```python
from build123d import *

# Parameters (mm, degrees)
F0_R     = 12.7
F1_DEPTH = 12.7
F3_R     = 4.7625
F3_R_2   = 2.7305
F4_DEPTH = 6.35


with BuildPart() as f1:
    # F0 (on Top) → F1 (new body)
    with BuildSketch(Plane.XY):
        Circle(F0_R)
    extrude(amount=F1_DEPTH)

    # F3 (on offset) → F4 (join)
    with BuildSketch(Plane.XY.offset(12.7)):
        with Locations((-5.399791, 5.753814)):
            Circle(F3_R)
        with Locations((-5.399791, 5.753814)):
            Circle(F3_R_2, mode=Mode.SUBTRACT)
        with Locations((-5.753814, -5.399791)):
            Circle(F3_R)
        with Locations((-5.753814, -5.399791)):
            Circle(F3_R_2, mode=Mode.SUBTRACT)
        with Locations((5.399791, -5.753814)):
            Circle(F3_R)
        with Locations((5.399791, -5.753814)):
            Circle(F3_R_2, mode=Mode.SUBTRACT)
        with Locations((5.753814, 5.399791)):
            Circle(F3_R)
        with Locations((5.753814, 5.399791)):
            Circle(F3_R_2, mode=Mode.SUBTRACT)
    extrude(amount=F4_DEPTH)


solid = f1.part
```
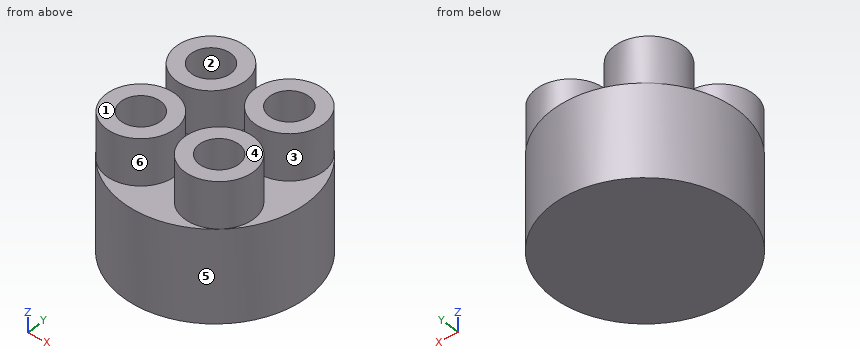
CAD build for the part. Positions are in the model's coordinates, mm. Face numbers are marked on the shaded views. A direction names the side the tool comes from. Coordinates: 2 decimals unless noted, no trailing zeros. Order: outer loops, then holes, each group sorted by start corner. A loop starts at its lowest first (then second) coordinate and runs counter-clockwise, first axis right, second up.
(1) Saw through at A-A, the plane x = -7.5. Write the cut outline in (y, z).
Solution:
outline: (-10.25, 0) - (10.25, 0) - (10.25, 12.7) - (10.03, 12.7) - (10.03, 19.05) - (7.5, 19.05) - (7.5, 12.7) - (4.01, 12.7) - (4.01, 19.05) - (1.48, 19.05) - (1.48, 12.7) - (-0.97, 12.7) - (-0.97, 19.05) - (-3.3, 19.05) - (-3.3, 12.7) - (-7.5, 12.7) - (-7.5, 19.05) - (-9.83, 19.05) - (-9.83, 12.7) - (-10.25, 12.7) - close
(2) Which spindle directions (+Z, -Z, +X, -X, +Y, -Y) get a long thin tool onto all of the face, cutting with end or side? Do the marked faces 1 and 2. Say none if no direction does.
Solution:
face 1: +Z, +X, -X, +Y, -Y
face 2: +Z
(3) Saw through at C-C, the plane z = 12.25. Write the cut outline in (x, y).
Solution:
outline: circle Ø25.4 at (0, 0)
(4) Mould opens along Y. For the marked faces 3, 4, 5 and 6 say: released by +Y, released by -Y, zero draft, split by the parting line, or undercut.
Solution:
face 3: undercut
face 4: zero draft
face 5: split by the parting line
face 6: undercut
(5) Saw through at B-B, the plane y = 9.5. Write the cut outline in (x, z).
Solution:
outline: (-8.43, 0) - (8.43, 0) - (8.43, 12.7) - (8.18, 12.7) - (8.18, 19.05) - (3.33, 19.05) - (3.33, 12.7) - (-2.46, 12.7) - (-2.46, 19.05) - (-8.34, 19.05) - (-8.34, 12.7) - (-8.43, 12.7) - close
(6) Pin check, flat tips, straight feed: pin 1 Ø8 at (x, z) = (-10, 3) entering from -Y; pin 2 Ø3 at (y, z) = (-9, 4.5) entering from -X; pin 3 Ø1.5 at (x, z) = (6.5, 3.5) entering from +Y. Stop position of each tip, or through.
Solution:
pin 1: stops at y = -11.19
pin 2: stops at x = -10.25
pin 3: stops at y = 11.32
(7) Drill centre lines: L1, parallel to Y at x = -6, z = 12.75; L2, parallel to Z at x = 8.5, y = 0.5; L3, parallel to Y at x = -2.5, z = 18. Where is each one in solid material? Low to high.
Solution:
L1: y = -10.16 to -8.12, -2.68 to -0.64, 1.03 to 3.09, 8.42 to 10.48
L2: z = 0 to 12.7
L3: y = -8.88 to -1.92, 1.98 to 9.53
(8) Saw through at D-D, the plane x = 9. Write the cut outline in (y, z), and give its area (3 significant figures).
Solution:
outline: (-8.96, 0) - (8.96, 0) - (8.96, 12.7) - (8.88, 12.7) - (8.88, 19.05) - (1.92, 19.05) - (1.92, 12.7) - (-2.64, 12.7) - (-2.64, 19.05) - (-8.87, 19.05) - (-8.87, 12.7) - (-8.96, 12.7) - close
area: 311 mm2
